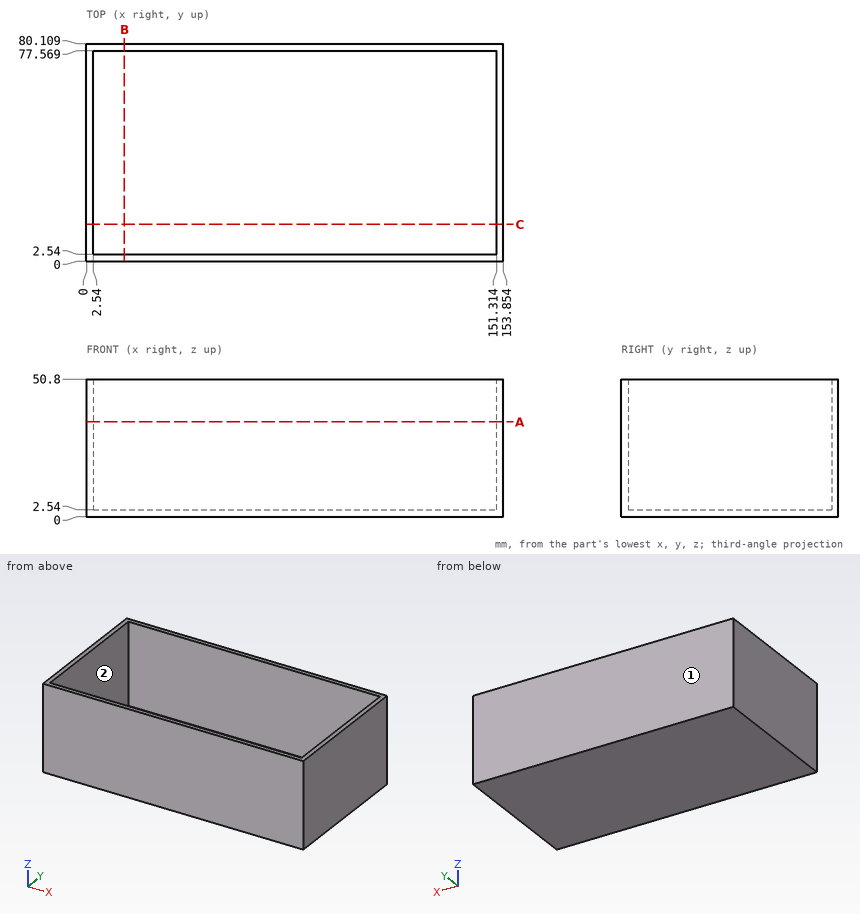
Study the drawing (mm; zero at the part's minimum x, y, z) and answer. A direction names the side the tool comes from. Coordinates: 2 decimals unless noted, no trailing zeros. Order: outer loops, then holes, each group sorted by start corner. A loop starts at its lowest first (then second) coordinate and runs counter-clockwise, first axis right, second up. Notation, with made-up numbers: M 23.5,88 L 42.5,88 A27 cw 42.5,117 Z; hole C -4.75,88 d4. An arc over 180 degrees is marked long. Answer as a JSON object with one key per item and string values. Group by question number.
1. Section B-B on x = 14 is taken. Write down the section's boundary in (y, z).
2. Straight lines are drawn through the part: line 1 (X direction, y = 71, z = 43.5); line 2 (Y direction, x = 47.5, z = 30); line 3 (Z direction, x = 70, y = 73). For each, find the intervals that lie inside material, in ascending order.
3. Section C-C on y = 13.5 is taken. Write down the section's boundary in (x, z), then the cut area to 3 significant figures.
4. A tool of negligible diameter and unlimited length cuts with its end or side. For the marked faces 1 and 2, from which of +Z, -Z, +X, -X, +Y, -Y can it reach the whole face along a straight path? Write none if from no direction.
5. Section A-A on z = 35 is taken. Write down the section's boundary in (x, y), then the cut area to 3 significant figures.
Values follow:
{
 "1": {"outline": "M 0,0 L 80.11,0 L 80.11,50.8 L 77.57,50.8 L 77.57,2.54 L 2.54,2.54 L 2.54,50.8 L 0,50.8 Z"},
 "2": {"line 1": "0 to 2.54, 151.31 to 153.85", "line 2": "0 to 2.54, 77.57 to 80.11", "line 3": "0 to 2.54"},
 "3": {"outline": "M 0,0 L 153.85,0 L 153.85,50.8 L 151.31,50.8 L 151.31,2.54 L 2.54,2.54 L 2.54,50.8 L 0,50.8 Z", "area": "636 mm2"},
 "4": {"face 1": "+Z, -Z, +X, -X, +Y", "face 2": "+Z"},
 "5": {"outline": "M 0,0 L 153.85,0 L 153.85,80.11 L 0,80.11 Z; hole M 2.54,2.54 L 151.31,2.54 L 151.31,77.57 L 2.54,77.57 Z", "area": "1,160 mm2"}
}
